```python
from build123d import *

# Parameters (mm, degrees)
SKETCH1_W           = 255
SKETCH1_H           = 200
SKETCH1_R           = 30
BOSS_EXTRUDE1_DEPTH = 5
SKETCH2_R           = 1
CUT_EXTRUDE1_DEPTH  = 28


with BuildPart() as part:
    # Sketch1 → Boss-Extrude1 (new body)
    with BuildSketch(Plane.XY):
        with Locations((127.5, 100)):
            Rectangle(SKETCH1_W, SKETCH1_H)
        with Locations((127.5, 100)):
            Circle(SKETCH1_R, mode=Mode.SUBTRACT)
    extrude(amount=BOSS_EXTRUDE1_DEPTH)

    # Sketch2 → Cut-Extrude1 (cut)
    with BuildSketch(Plane.XY):
        with Locations(Location((61, 100, 0), (0, 0, 180))):
            Circle(SKETCH2_R)
        with Locations(Location((127.5, 166.5, 0), (0, 0, 180))):
            Circle(SKETCH2_R)
        with Locations(Location((194, 100, 0), (0, 0, 180))):
            Circle(SKETCH2_R)
        with Locations(Location((127.5, 33.5, 0), (0, 0, 180))):
            Circle(SKETCH2_R)
    extrude(amount=CUT_EXTRUDE1_DEPTH, mode=Mode.SUBTRACT)


solid = part.part
```
Design review of the part built by this model. Coordinates are the model's own, in mm. Give positions to 0.01 mm unless a question says otherwise; leave off trailing zeros. Write each loop counter-clockwise with the first axis right and the second up, starting at its lowest first coordinate (ties: lowest second). Pieces come first, ordered by that corner, then holes. Notation, with made-up numbers: (-26.75, 17) -> (24.25, 17) arc R22 cw to (24.25, 30) -> close; hole circle Ø2 at (33, 74). An arc over 180 degrees is marked (long way). Answer in a Markdown table with one row per item.
(1) Mouldability with a two-part tool opening along X and no side actions: class faces 1 (the flat face through (0, 99, 2)), 2 (the cylindrical face through (105.389, 120.275, 2.465)), 3 (the flat face through (255, 99, 2)), 4 (the flat face through (97, 101, 0)) as +X half, -X half, draft (parallel to the pull), parting line (faces both ways), or undercut.
Results:
| item | result |
|---|---|
| face 1 | -X half |
| face 2 | undercut |
| face 3 | +X half |
| face 4 | draft |
(2) Consider section B-B (x = 102). State the section outline as (y, z) points, then the cut area to 3 significant figures.
Results:
| item | result |
|---|---|
| outline | (0, 0) -> (84.2, 0) -> (84.2, 5) -> (0, 5) -> close; (115.8, 0) -> (200, 0) -> (200, 5) -> (115.8, 5) -> close |
| area | 842 mm2 |
(3) Clearance check with flat-ended pins moving along their axes: pin 1 (3 mm diameter, centred on x = 127.5, y = 33.5, fed in from -Z); pin 2 (1.8 mm diameter, centred on x = 61, y = 100, fed in from -Z). State where each tip first meets the part, or that it passes through.
Results:
| item | result |
|---|---|
| pin 1 | z = 0 |
| pin 2 | through |
(4) Consider section C-C (x = 137). State the section outline as (y, z) points, then the cut area to 3 significant figures.
Results:
| item | result |
|---|---|
| outline | (0, 0) -> (71.54, 0) -> (71.54, 5) -> (0, 5) -> close; (128.46, 0) -> (200, 0) -> (200, 5) -> (128.46, 5) -> close |
| area | 715 mm2 |
(5) Consider section A-A (z = 3.7). State the section outline as (x, y) points.
Results:
| item | result |
|---|---|
| outline | (0, 0) -> (255, 0) -> (255, 200) -> (0, 200) -> close; hole circle Ø2 at (61, 100); hole circle Ø60 at (127.5, 100); hole circle Ø2 at (127.5, 33.5); hole circle Ø2 at (127.5, 166.5); hole circle Ø2 at (194, 100) |
(6) To check wall thickness, follow probe 1 along Y at (x, z) = (127.5, 3.3); probe 2 along Y at (x, z) = (194, 2.05); probe 3 along X at (y, z) = (124, 1.15). State the ranges of each line that lie inside material, in increasing order.
Results:
| item | result |
|---|---|
| probe 1 | 0 to 32.5, 34.5 to 70, 130 to 165.5, 167.5 to 200 |
| probe 2 | 0 to 99, 101 to 200 |
| probe 3 | 0 to 109.5, 145.5 to 255 |
